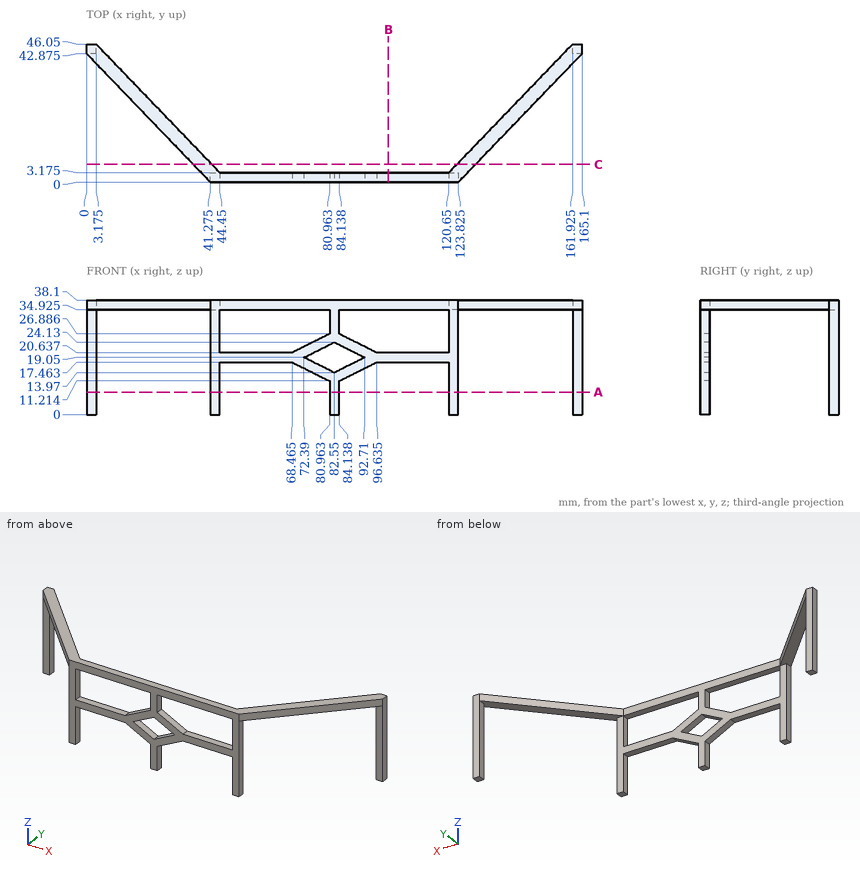
Here's the drawing with two shaded views (mm, measured from the low corner). I have some questions. Coordinates: 2 decimals unless noted, no trailing zeros. Write each loop counter-clockwise with the first axis right and the second up, starting at its lowest first coordinate (ties: lowest second). Pieces come first, ordered by that corner, then holes. Notation, with made-up numbers: (69, 57.5) -> (127, 57.5) arc R12 cw to (127, 62.5) -> close; hole circle Ø10 at (-4, 12.5). An arc over 180 degrees is marked (long way). Use a Markdown table: item, result. Add a question column.
(1) I'm going to push flat-ended pins straight in: P1, Ø2.5, axis at x = 70, y = 1, coming from the -Z side; P2, Ø12, axis at x = 140, z = 26.5, coming from the +Y side; P3, Ø13.5, axis at x = 29, y = 18.5, coming from the -Z side (1 decimal); P4, Ø1, axis at x = 109, y = 1, coming from the -Z side. Where does each tip first touch, or does it pass through?
(2) Please list where these lines run through material, in increasing order: line 1 (Z direction, x = 145, y = 28) (1 decimal); line 2 (Y direction, x = 85, z = 36) (1 decimal); line 3 (X direction, y = 35.5, z = 36).
(3) If we section it at C-C, the plane y = 6: Write out the boundary of the cut face in (x, z) (1 decimal).
(4) If we section it at A-A, the plane z = 7.5: State how many separate pieces and enclosed holes the cut face has.
(5) If we section it at B-B, the plane x = 100.5: Write out the boundary of the cut face in (y, z) (1 decimal).
Outcome:
| question | item | result |
|---|---|---|
| 1 | P1 | stops at z = 16.07 |
| 1 | P2 | passes through |
| 1 | P3 | stops at z = 34.9 |
| 1 | P4 | stops at z = 17.46 |
| 2 | line 1 | z = 34.9 to 38.1 |
| 2 | line 2 | y = 0 to 3.2 |
| 2 | line 3 | x = 7.1 to 13.33, 151.77 to 158 |
| 3 | outline | (35.5, 34.9) -> (41.7, 34.9) -> (41.7, 38.1) -> (35.5, 38.1) -> close; (123.4, 34.9) -> (129.6, 34.9) -> (129.6, 38.1) -> (123.4, 38.1) -> close |
| 4 | separate pieces | 5 |
| 4 | enclosed holes | 0 |
| 5 | outline | (0, 17.5) -> (3.2, 17.5) -> (3.2, 20.6) -> (0, 20.6) -> close; (0, 34.9) -> (3.2, 34.9) -> (3.2, 38.1) -> (0, 38.1) -> close |
